The listing builds one solid part. Answer for the finished solid, in the listing's coordinates (mm). A direction names the side the tool comes from. Round coordinates to 2 decimals unless told otherwise and drop trailing zeros. Write each loop counter-clockwise with the first axis right and the second up, starting at its lowest first coordinate (ties: lowest second). Pieces come first, ordered by that corner, then holes.
(1) Find the intervals of material crossed by probe 1 along Z at (x, y) = (1, 1.5); probe 2 along Z at (x, y) = (-7, 2); probe 3 along Y at (x, z) = (-13.5, 20), in increasing order.
(2) Each of these flat-tipped pins is pushed along its axis until it touches: pin 1 Ø6 at (x, z) = (1.5, 9.5) entering from +Y; pin 2 Ø4 at (y, z) = (5.5, 4) entering from -X; pin 3 Ø12 at (y, z) = (11, -4.5) entering from -X; pin 4 Ø12 at (y, z) = (20.5, 11) entering from +X. Where does it stop, or does it pass through?
(3) A cutting plane is placed at A-A, the plane x = 0. Give the vertices of the cut face in (y, z), and give its area (3 significant figures).
(4) For faces 4 (the face through (0, 4, 11)), 5 (the face through (-7.84, 2.46, 2.72)), 6 (the face through (-16, 4, -4.497)), determine the directions among +Z, -Z, +X, -X, +Y, -Y from which every point of the face is accessible in a straight line to the end or side of a thin tool.
(5) The mould has two halves that part along Z. Classify faces 1 (the face through (-3, 16, 0)), 2 (the face through (7.84, 2.46, 2.72)), 3 (the face through (19, 4, -4.497)): +Z half, -Z half, draft (parallel to the pull), parting line (faces both ways), or undercut.
(6) A cutting plane is placed at B-B, the plane z = 9. Give the number of separate pieces and of enclosed holes in the cut face, and give its area (3 significant figures).
Autodesk Inventor part; units mm, degrees
ref_plane "XZ Plane" through (0, 0, 0) normal (0, 1, 0) x (-1, 0, 0)
ref_plane "XY Plane" through (0, 0, 0) normal (0, 0, 1) x (1, 0, 0)
sketch "Skizze1" plane through (0, 0, 0) normal (0, 1, 0) x (-1, 0, 0)
  circle A0 centre (0, 0) radius 27.5
  circle A1 centre (0, 0) radius 22.5
  circle A2 centre (0, 0) radius 3.5
  line L0 (45.7225, 0) -> (-63.662, 0) construction
  line L1 (0, 78.2374) -> (0, -78.2374) construction
  circle A3 centre (15, 0) radius 2
  circle A4 centre (-15, 0) radius 2
  line L2 (0, 3.5) -> (15.1977, 1.9902)
  line L3 (15.1977, -1.9902) -> (0, -3.5)
  line L4 (-14.8023, -1.9902) -> (0, -3.5)
  line L5 (0, 3.5) -> (-15.1977, 1.9902)
  circle A5 centre (0, 0) radius 11
  line L6 (10.0387, 4.4973) -> (22.046, 4.4973)
  line L7 (-10.0387, 4.4973) -> (-22.046, 4.4973)
  line L8 (10.0387, -4.4973) -> (22.046, -4.4973)
  line L9 (-10.0387, -4.4973) -> (-22.046, -4.4973)
  point P0 (27.1298, 4.4973)
  point P1 (-27.023, -5.1)
  point P2 (13.75, -23.8157)
  point P3 (-13.75, 23.8157)
  point P4 (-0.6886, 3.4316)
  point P5 (0.6886, 3.4316)
  point P6 (0.6886, -3.4316)
  point P7 (-0.7066, -3.4279)
  dimension "d0" = 55
  dimension "d1" = 45
  dimension "d2" = 7
  dimension "d3" = 4
  dimension "d4" = 4
  dimension "d5" = 15
  dimension "d6" = 22
ref_plane "Arbeitsebene1" through (0, 3.7, 0) normal (0, 1, 0) x (1, 0, 0)
extrude "Extrusion3" add sketch "Skizze1" along normal blind 8 contours A0 | A1 L8 A5 L3 A3 L2 L6 | L7 A5 L5 A4 L4 L9 A1 | A5 L2 A2 L5 | A5 L4 A2 L3
sketch "Skizze3" plane through (0, 8, 0) normal (0, 1, 0) x (1, 0, 0)
  arc A0 (22.046, 4.4973) -> (-22.046, 4.4973) centre (0, 0) ccw
  arc A1 (-22.046, -4.4973) -> (22.046, -4.4973) centre (0, 0) ccw
  line L0 (-22.046, 4.4973) -> (22.046, 4.4973)
  line L1 (22.046, 4.4973) -> (22.046, -4.4973)
  line L2 (22.046, -4.4973) -> (-22.046, -4.4973)
  line L3 (-22.046, -4.4973) -> (-22.046, 4.4973)
extrude "Extrusion4" add sketch "Skizze3" against normal blind 3 contours L1 L2 L3 L0
sketch "Skizze7" plane through (0, 8, 0) normal (0, 1, 0) x (1, 0, 0)
  arc A0 (22.046, 4.4973) -> (-22.046, 4.4973) centre (0, 0) ccw
  line L0 (-22.046, 4.4973) -> (-27.1298, 4.4973)
  circle A1 centre (0, 0) radius 27.5
  line L1 (22.046, 4.4973) -> (10.0387, 4.4973)
  line L2 (22.046, 4.4973) -> (27.1412, 4.4973)
  line L3 (27.1412, 4.4973) -> (9.9712, 4.4973)
  arc A2 (10.0387, 4.4973) -> (-10.0387, 4.4973) centre (0, 0) ccw
  line L4 (-22.046, 4.4973) -> (-10.0387, 4.4973)
  circle A3 centre (0, 0) radius 11
  circle A4 centre (0, 0) radius 27.5
  point P0 (27.1298, 4.4973)
extrude "Extrusion8" cut sketch "Skizze7" against normal blind 10 contours L1 A2 L4 A0 | A0 L0 A1 L2
fillet "Rundung8" radius 6 1 edges at (-27.1298, 4, -4.4973)
fillet "Rundung9" radius 2 6 edges at (-25.8358, 0, -2.589) (-15.743, 0, -4.4973) (3.2133, 0, 27.3116) (-25.8358, 8, -2.589) (-15.743, 8, -4.4973) (3.2133, 8, 27.3116)
sketch "Skizze9" plane through (0, 8, 0) normal (0, 1, 0) x (1, 0, 0)
  circle A0 centre (0, 0) radius 3
  dimension "d47" = 6
extrude "Extrusion9" add sketch "Skizze9" along normal blind 15
fillet "Rundung10" radius 2 3 edges at (10.0387, 4, 4.4973) (10.0387, 4, -4.4973) (-10.0387, 4, 4.4973)
fillet "Rundung11" radius 2 1 edges at (-3, 8, 0)
ref_plane "Arbeitsebene4" through (0, 0, 0) normal (1, 0, 0) x (0, 1, 0)
sketch "Skizze10" plane through (27.1298, 2, -4.4973) normal (0, 0, -1) x (-1, 0, 0)
  line L0 (0, 0) -> (0, 4)
  line L1 (0, 2) -> (17.4598, 2)
  circle A0 centre (6, 2) radius 3
  point P0 (27.1298, -2)
  dimension "d53" = 6
  dimension "d54" = 6
sketch "Skizze11" plane through (0, 0, 0) normal (1, 0, 0) x (0, 1, 0)
  line L0 (4, -48.7659) -> (4, 34.6929) construction
  line L1 (8, -11) -> (8, -2.4973) construction
  circle A0 centre (4, -19) radius 2
  point P0 (0, 0)
  point P1 (8, -5.4977)
  dimension "d55" = 4
  dimension "d56" = 4
  dimension "d57" = 8
sketch "Skizze12" plane through (0, 3.7, 0) normal (0, 1, 0) x (1, 0, 0)
  arc A0 (-25.4376, -1.7823) -> (25.1003, 4.4973) centre (0, 0) ccw
  spline S0 degree 2 poles (25.1003, 4.4973) (21.7392, 19.3697) (0, 19.7453) knots 0 0 0 1 1 1
  point P0 (18.4599, 14.8701)
properties part number "_3D-Druck"
Solutions:
1. probe 1: z = -10.95 to -3.4, 3.4 to 10.95, 22.48 to 27.42
1. probe 2: z = -8.49 to -2.8, 2.8 to 8.49, 21.38 to 26.59
1. probe 3: y = 0 to 8
2. pin 1: stops at y = 8
2. pin 2: stops at x = -27.43
2. pin 3: stops at x = -27.03
2. pin 4: passes through
3. outline: (0, -11) - (8, -11) - (8, -5) arc R2 cw to (10, -3) - (23, -3) - (23, 3) - (10, 3) arc R2 cw to (8, 5) - (8, 11) - (0, 11) - (0, 3.5) - (5, 3.5) - (5, -3.5) - (0, -3.5) - close; (0, 22.5) - (8, 22.5) - (8, 25.5) arc R2 ccw to (6, 27.5) - (2, 27.5) arc R2 ccw to (0, 25.5) - close
3. area: 271 mm2
4. face 4: +Y, -Y
4. face 5: -Y
4. face 6: -Z, -X, +Y, -Y
5. face 1: parting line
5. face 2: undercut
5. face 3: -Z half
6. separate pieces: 3
6. enclosed holes: 0
6. area: 183 mm2
